Can you work these out from the drawing? Everything is in mm from the part's minimum corner. A direction names the side the tool comes from. Round coordinates to 2 decimals unless told otherwise and drop trailing zeros. Write each loop counter-clockwise with the first axis right and the second up, starting at its lowest first coordinate (ties: lowest second). Pieces come first, ordered by that corner, then holes.
Q1. We'd pull the mould along Z, two halves only. Please class the marked faces 1, 2 and 3: +Z half, -Z half, draft (parallel to the pull), parting line (faces both ways), or undercut.
Q2. If we section it at A-A (z = 7): Please give me the cut outline in (x, y), plus the area to 3 significant figures.
Q3. I'm going to push flat-ended pins straight in: pin 1 Ø3 at (x, z) = (37, 7) entering from +Y; pin 2 Ø5.5 at (x, z) = (34, 7.5) entering from +Y; pin 3 Ø3 at (y, z) = (15, 11.5) entering from -X; pin 4 Ø1.5 at (x, y) = (17.5, 30) entering from -Z. Where does each tip first touch, or does it pass through?
Q4. For the marked faces 4, 5 and 6, which set-ups out of +Z, -Z, +X, -X, +Y, -Y let a thin tool reach every point of the face, with its end or its side?
Q5. If we section it at D-D (z = 12.5): Please give me the cut outline in (x, y), plus the area to 3 significant figures.
Q6. If we section it at C-C (x = 3): Please give me the cut outline in (y, z), plus the area to 3 significant figures.
Q7. If we section it at B-B (y = 23): Please give me the cut outline in (x, z), plus the area to 3 significant figures.
Q8. Please list where these lines run through material, in increasing order: line 1 along Z through (x, y) = (5, 1.75); line 2 along Y through (x, z) = (21, 5); line 3 along X through (y, z) = (9, 12.5).
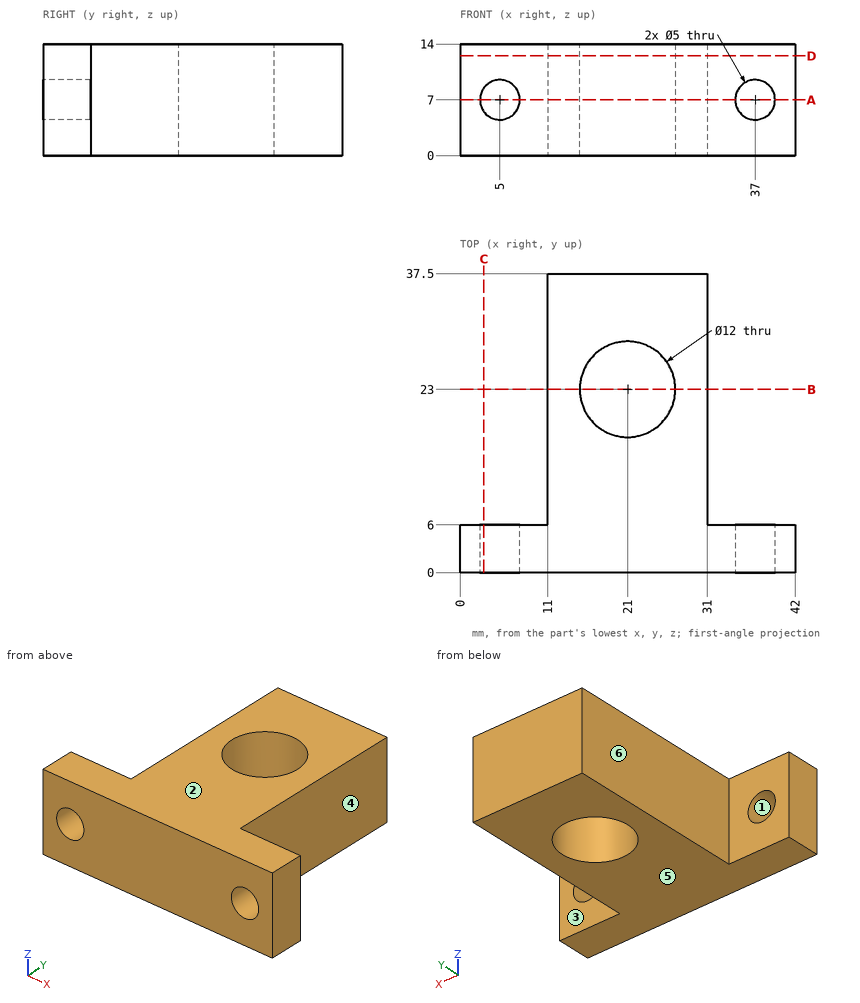
A:
1. face 1: undercut
1. face 2: +Z half
1. face 3: draft
2. outline: (0, 0) - (2.5, 0) - (2.5, 6) - (0, 6) - close; (7.5, 0) - (34.5, 0) - (34.5, 6) - (31, 6) - (31, 37.5) - (11, 37.5) - (11, 6) - (7.5, 6) - close; (39.5, 0) - (42, 0) - (42, 6) - (39.5, 6) - close; hole circle Ø12 at (21, 23)
2. area: 709 mm2
3. pin 1: passes through
3. pin 2: stops at y = 6
3. pin 3: stops at x = 11
3. pin 4: stops at z = 0
4. face 4: +Z, -Z, +X, +Y
4. face 5: -Z, +X, -X, +Y, -Y
4. face 6: +Z, -Z, -X, +Y
5. outline: (0, 0) - (42, 0) - (42, 6) - (31, 6) - (31, 37.5) - (11, 37.5) - (11, 6) - (0, 6) - close; hole circle Ø12 at (21, 23)
5. area: 769 mm2
6. outline: (0, 0) - (6, 0) - (6, 5.5) - (0, 5.5) - close; (0, 8.5) - (6, 8.5) - (6, 14) - (0, 14) - close
6. area: 66.0 mm2
7. outline: (11, 0) - (15, 0) - (15, 14) - (11, 14) - close; (27, 0) - (31, 0) - (31, 14) - (27, 14) - close
7. area: 112 mm2
8. line 1: z = 0 to 4.5, 9.5 to 14
8. line 2: y = 0 to 17, 29 to 37.5
8. line 3: x = 11 to 31
